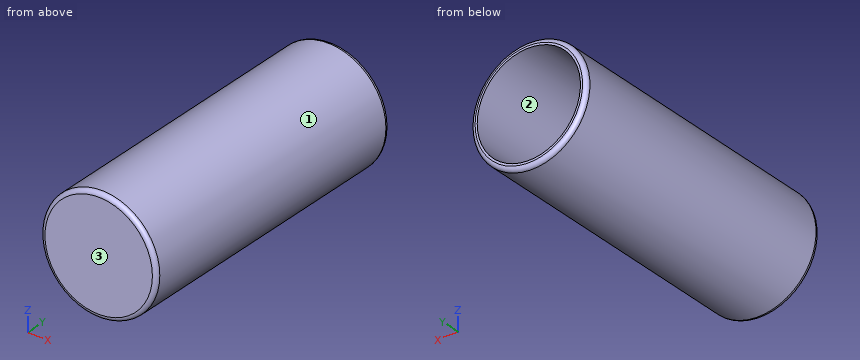
from build123d import *

# Parameters (mm, degrees)
SKETCH1_R           = 13.75
BOSS_EXTRUDE1_DEPTH = 72.5
SKETCH2_R           = 12.25
CUT_EXTRUDE1_DEPTH  = 71
FILLET1_R           = 1


with BuildPart() as part:
    # Sketch1 → Boss-Extrude1 (new body)
    with BuildSketch(Plane(origin=(0, 0, 0), x_dir=(1, 0, 0), z_dir=(0, 1, 0))):
        Circle(SKETCH1_R)
    extrude(amount=BOSS_EXTRUDE1_DEPTH)

    # Sketch2 → Cut-Extrude1 (cut)
    with BuildSketch(Plane(origin=(0, 72.5, 0), x_dir=(1, 0, 0), z_dir=(0, 1, 0))):
        Circle(SKETCH2_R)
    extrude(amount=-CUT_EXTRUDE1_DEPTH, mode=Mode.SUBTRACT)

    # Fillet1
    fillet1_edges = [part.edges().sort_by_distance(p)[0] for p in [
        (-13.75, 0, 0),
        (-13.75, 72.5, 0),
    ]]
    fillet(fillet1_edges, radius=FILLET1_R)


solid = part.part
Model file for the job. Use its own axes, mm. Face numbers are marked on the shaded views. Round coordinates to 2 decimals unless told otherwise and drop trailing zeros. Order: outer loops, then holes, each group sorted by start corner. A loop starts at its lowest first (then second) coordinate and runs counter-clockwise, first axis right, second up. Notation, with made-up numbers: M 2.5,-1 L 25.5,-1 A21 cw 25.5,24 Z; hole C 38.5,42.25 d7. An arc over 180 degrees is marked long. Write each question's results on one line, items separated by ' | '. Start each with the question number.
(1) Saw through at C-C, the plane y = 22. Give the cut face in (x, z).
(2) Two-plate mould, pull along Z, no slides. Class the marked faces 1, 2 and 3: pulls with the +Z half, pulls with the -Z half, needs draft (parallel to the pull), parting line crosses it, or undercut.
(3) Probe probe 1 along X at (y, z) = (48.5, 0); probe 2 along Z at (x, y) = (0.5, 53.5); probe 3 along Y at (x, z) = (-1.5, -1). List the from-to ranges inside material, lowest first. Write a range as from..to.
(4) Saw through at B-B, the plane z = 0. Give the cut face in (x, y).
(5) Drop flat-ended pins along their axis: pin 1 (1 mm diameter, centred on x = -10.5, z = 5, fed in from +Y); pin 2 (3 mm diameter, centred on y = 59.5, z = 6, fed in from -X); pin 3 (1.5 mm diameter, centred on y = 53, z = 8.5, fed in from -X). Give the stop position or say it passes through.
(6) Saw through at A-A, the plane x = 0. Give the cut face in (y, z).
Established:
1) outline: C 0,0 d27.5; hole C 0,0 d24.5
2) face 1: parting line crosses it | face 2: undercut | face 3: needs draft
3) probe 1: x = -13.75..-12.25, 12.25..13.75 | probe 2: z = -13.74..-12.24, 12.24..13.74 | probe 3: y = 0..1.5
4) outline: M -13.75,1 A1 ccw -12.75,0 L 12.75,0 A1 ccw 13.75,1 L 13.75,71.5 A1 ccw 12.75,72.5 L 12.25,72.5 L 12.25,1.5 L -12.25,1.5 L -12.25,72.5 L -12.75,72.5 A1 ccw -13.75,71.5 Z
5) pin 1: stops at y = 1.5 | pin 2: stops at x = -12.99 | pin 3: stops at x = -11.36
6) outline: M 0,-12.75 A1 ccw 1,-13.75 L 71.5,-13.75 A1 ccw 72.5,-12.75 L 72.5,-12.25 L 1.5,-12.25 L 1.5,12.25 L 72.5,12.25 L 72.5,12.75 A1 ccw 71.5,13.75 L 1,13.75 A1 ccw 0,12.75 Z
